The model under review builds one solid part; all positions refer to its coordinate system, in mm. Round coordinates to 2 decimals unless told otherwise and drop trailing zeros. Write each loop counter-clockwise with the first axis right and the second up, starting at its lowest first coordinate (ties: lowest second). Pieces come first, ordered by that corner, then holes. Notation, with made-up numbers: (39.25, 48) -> (68.25, 48) arc R25 cw to (68.25, 80) -> close; hole circle Ø5 at (16.5, 0). An arc over 180 degrees is marked (long way). Answer as a JSON object with one key per item and string values. Group by question number.
1) We need section C-C, the plane z = 29. Write out the cut boundary in (x, y).
2) Mouldability with a two-part tool opening along X and no side actions: class faces 1 (the conical face through (63.062, -13.925, 33.25)), 2 (the flat face through (92.276, -0.117, 30.428)), 3 (the conical face through (-10.2, -7.8, 23)) as pulls with the +X half, pulls with the -X half, needs draft (parallel to the pull), parting line crosses it, or undercut.
3) To check wall thickness, follow probe 1 along Y at (x, z) = (0, -47); probe 2 along Z at (x, y) = (120.5, 17.5); probe 3 along X at (y, z) = (3, -14). State the ranges of each line that lie inside material, in increasing order. Write a range as [from, to].
4) Insertion check: pin 1 Ø3 at (x, y) = (76, -15) entering from -Z; pin 2 Ø13.5 at (x, y) = (94.5, -4) entering from +Z; pin 3 Ø10 at (x, y) = (45.5, 14.5) entering from +Z; pin 4 Ø12 at (x, y) = (-5.5, 0) entering from +Z. Each pin has a flat end and moves straight along its axis. Give the tip position at first contact, or say it passes through.
5) We need section A-A, the plane z = -28. Write out the cut boundary in (x, y).
6) We need section B-B, the plane z = 15. Write out the cut boundary in (x, y).
from build123d import *

# Parameters (mm, degrees)
F0_R     = 12.7
F1_DEPTH = 25.4
F2_DEPTH = 76.2
F5_DEPTH = 12.7
F6_SIZE  = 12.69999
F7_SIZE  = 2.54
F8_SIZE  = 2.54
F9_SIZE  = 2.54


# Not quite as in the source:
# - a fillet or chamfer is up to 0.001 mm smaller than in the source, because OpenCascade refuses the exact size


with BuildPart() as f1:
    # F0 (on Top) → F1 (new body)
    with BuildSketch(Plane.XY):
        with BuildLine():
            ThreePointArc((0, -25.4), (17.9605122421, -17.9605122421), (25.4, 0))
            ThreePointArc((25.4, 0), (17.9605122421, 17.9605122421), (0, 25.4))
            ThreePointArc((0, 25.4), (-25.4, 0), (0, -25.4))
        make_face()
        Circle(F0_R, mode=Mode.SUBTRACT)
        with BuildLine():
            ThreePointArc((0, 25.4), (17.9605122421, 17.9605122421), (25.4, 0))
            ThreePointArc((25.4, 0), (17.9605122421, -17.9605122421), (0, -25.4))
            Line((0, -25.4), (127, -25.4))
            ThreePointArc((127, -25.4), (101.6, 0), (127, 25.4))
            Line((127, 25.4), (0, 25.4))
        make_face()
        with BuildLine():
            ThreePointArc((152.4, 0), (144.9605122421, 17.9605122421), (127, 25.4))
            ThreePointArc((127, 25.4), (101.6, 0), (127, -25.4))
            ThreePointArc((127, -25.4), (144.9605122421, -17.9605122421), (152.4, 0))
        make_face()
        with Locations((127, 0)):
            Circle(F0_R, mode=Mode.SUBTRACT)
    extrude(amount=F1_DEPTH)

    # F0 (on Top) → F2 (join)
    with BuildSketch(Plane.XY):
        with BuildLine():
            ThreePointArc((0, -25.4), (17.9605122421, -17.9605122421), (25.4, 0))
            ThreePointArc((25.4, 0), (17.9605122421, 17.9605122421), (0, 25.4))
            ThreePointArc((0, 25.4), (-25.4, 0), (0, -25.4))
        make_face()
        Circle(F0_R, mode=Mode.SUBTRACT)
        with BuildLine():
            ThreePointArc((152.4, 0), (144.9605122421, 17.9605122421), (127, 25.4))
            ThreePointArc((127, 25.4), (101.6, 0), (127, -25.4))
            ThreePointArc((127, -25.4), (144.9605122421, -17.9605122421), (152.4, 0))
        make_face()
        with Locations((127, 0)):
            Circle(F0_R, mode=Mode.SUBTRACT)
    extrude(amount=-F2_DEPTH)

    # F4 (on face) → F5 (join)
    with BuildSketch(Plane.XY.offset(25.4)):
        with BuildLine():
            ThreePointArc((29.6961453219, -8.3886324314), (63.5, -21.7770315987), (97.3038546781, -8.3886324314))
            Line((97.3038546781, -8.3886324314), (97.3038546781, 8.3886324314))
            ThreePointArc((97.3038546781, 8.3886324314), (63.5, 21.7770315987), (29.6961453219, 8.3886324314))
            Line((29.6961453219, 8.3886324314), (29.6961453219, -8.3886324314))
        make_face()
    extrude(amount=F5_DEPTH)

    # F6 (size 12.7 in the source; OpenCascade refuses exactly that, so slightly less here)
    f6_edges = [f1.edges().sort_by_distance(p)[0] for p in [
        (63.5, -21.777032, 38.1),
        (97.303855, 0, 38.1),
        (63.5, 21.777032, 38.1),
        (29.696145, 0, 38.1),
    ]]
    chamfer(f6_edges, length=F6_SIZE)

    # F7
    f7_edges = [f1.edges().sort_by_distance(p)[0] for p in [
        (114.3, 0, 25.4),
        (-12.7, 0, 25.4),
    ]]
    chamfer(f7_edges, length=F7_SIZE)

    # F8
    f8_edges = [f1.edges().sort_by_distance(p)[0] for p in [
        (114.3, 0, -76.2),
        (127, -25.4, -76.2),
        (-25.4, 0, -76.2),
        (-12.7, 0, -76.2),
    ]]
    chamfer(f8_edges, length=F8_SIZE)

    # F9
    f9_edges = [f1.edges().sort_by_distance(p)[0] for p in [
        (63.5, -25.4, 25.4),
    ]]
    chamfer(f9_edges, length=F9_SIZE)


solid = f1.part
Here are the results:
{
 "1": {"outline": "(33.3, -6.8) arc R45.77 ccw to (93.7, -6.8) -> (93.7, 6.8) arc R45.77 ccw to (33.3, 6.8) -> close"},
 "2": {"face 1": "parting line crosses it", "face 2": "pulls with the +X half", "face 3": "undercut"},
 "3": {"probe 1": "y = [-25.4, -12.7], [12.7, 25.4]", "probe 2": "z = [-76.2, 25.4]", "probe 3": "x = [-25.22, -12.34], [12.34, 25.22], [101.78, 114.66], [139.34, 152.22]"},
 "4": {"pin 1": "stops at z = 0", "pin 2": "stops at z = 34.95", "pin 3": "stops at z = 33.99", "pin 4": "passes through"},
 "5": {"outline": "circle Ø50.8 at (0, 0); circle Ø50.8 at (127, 0); hole circle Ø25.4 at (0, 0); hole circle Ø25.4 at (127, 0)"},
 "6": {"outline": "(0, -25.4) -> (127, -25.4) arc R25.4 ccw to (127, 25.4) -> (0, 25.4) arc R25.4 ccw to start; hole circle Ø25.4 at (0, 0); hole circle Ø25.4 at (127, 0)"}
}
